Build history of the part. All positions in model axes, mm. A direction names the side the tool comes from. Round coordinates to 2 decimals unless told otherwise and drop trailing zeros. Write each loop counter-clockwise with the first axis right and the second up, starting at its lowest first coordinate (ties: lowest second). Pieces come first, ordered by that corner, then holes. Notation, with made-up numbers: (-15, 26.25) -> (6, 26.25) arc R23 cw to (6, 36.25) -> close; hole circle Ø5 at (12, 53). An arc over 180 degrees is marked (long way). Answer in a Markdown table with one row per item. Add a question column.
from build123d import *

# Parameters (mm, degrees)
F0_W     = 43
F0_H     = 50
F0_R     = 16
F1_DEPTH = 2
F2_W     = 43
F2_H     = 2
F3_DEPTH = 20
F5_D     = 5


with BuildPart() as f1:
    # F0 (on Front) → F1 (new body)
    with BuildSketch(Plane.XZ):
        Rectangle(F0_W, F0_H)
        Circle(F0_R, mode=Mode.SUBTRACT)
    extrude(amount=F1_DEPTH)

    # F2 (on face) → F3 (join)
    with BuildSketch(Plane.XZ.offset(2)):
        with Locations((0, -24)):
            Rectangle(F2_W, F2_H)
    extrude(amount=F3_DEPTH)

    # F5 (through all)
    with Locations(Plane(origin=(0, 0, -25), x_dir=(1, 0, 0), z_dir=(0, 0, -1))):
        with Locations((-11.5, 12), (11.5, 12)):
            Hole(F5_D / 2)


solid = f1.part
(1) Saw through at B-B (z = -1). List the corners of the cut face in (x, y), plus the area to 3 significant figures.
(2) Probe line 1 along X through (y, z) = (-12, -23.5); line 2 along Y through (x, z) = (11.5, -24.4); line 3 along Y through (x, z) = (-3, 21). List the from-to ranges inside material, lowest first.
(3) Which spindle directions (+Z, -Z, +X, -X, +Y, -Y) get a long thin tool onto all of the face, cutting with end or side? Do faces 1 (the face through (0, -12, -23)), 2 (the face through (0, 0, 17)). Say none if no direction does.
(4) Saw through at A-A (y = -13.5). List the corners of the cut face in (x, z).
(5) Drop flat-ended pins along their axis: P1, Ø1.5, axis at x = -7, y = -12, coming from the +Z side; P2, Ø10, axis at x = -1.5, z = 18, coming from the -Y side. Give the stop position or say it passes through.
(6) Mould opens along X. For faces 3 (the face through (-21.5, -1, -8)), 4 (the face through (21.5, -1, -8)), 5 (the face through (-10.96, -9.56, -23.99)), 6 (the face through (0, -22, -24)) say: pulls with the +X half, pulls with the -X half, needs draft (parallel to the pull), parting line crosses it, or undercut.
(7) Saw through at D-D (x = 7). List the corners of the cut face in (y, z), plus the area to 4 significant figures.
(8) Saw through at C-C (x = -11.5). List the corners of the cut face in (y, z).
Answer sheet:
| question | item | result |
|---|---|---|
| 1 | outline | (-21.5, -2) -> (-15.97, -2) -> (-15.97, 0) -> (-21.5, 0) -> close; (15.97, -2) -> (21.5, -2) -> (21.5, 0) -> (15.97, 0) -> close |
| 1 | area | 22.1 mm² |
| 2 | line 1 | x = -21.5 to -14, -9 to 9, 14 to 21.5 |
| 2 | line 2 | y = -22 to -14.5, -9.5 to 0 |
| 2 | line 3 | y = -2 to 0 |
| 3 | face 1 | +Z, +X, -X, -Y |
| 3 | face 2 | +Z, -Z, +X, -X, +Y |
| 4 | outline | (-21.5, -25) -> (-13.5, -25) -> (-13.5, -23) -> (-21.5, -23) -> close; (-9.5, -25) -> (9.5, -25) -> (9.5, -23) -> (-9.5, -23) -> close; (13.5, -25) -> (21.5, -25) -> (21.5, -23) -> (13.5, -23) -> close |
| 5 | P1 | stops at z = -23 |
| 5 | P2 | stops at y = -2 |
| 6 | face 3 | pulls with the -X half |
| 6 | face 4 | pulls with the +X half |
| 6 | face 5 | undercut |
| 6 | face 6 | needs draft |
| 7 | outline | (-22, -25) -> (0, -25) -> (0, -14.39) -> (-2, -14.39) -> (-2, -23) -> (-22, -23) -> close; (-2, 14.39) -> (0, 14.39) -> (0, 25) -> (-2, 25) -> close |
| 7 | area | 82.45 mm² |
| 8 | outline | (-22, -25) -> (-14.5, -25) -> (-14.5, -23) -> (-22, -23) -> close; (-9.5, -25) -> (0, -25) -> (0, -11.12) -> (-2, -11.12) -> (-2, -23) -> (-9.5, -23) -> close; (-2, 11.12) -> (0, 11.12) -> (0, 25) -> (-2, 25) -> close |
